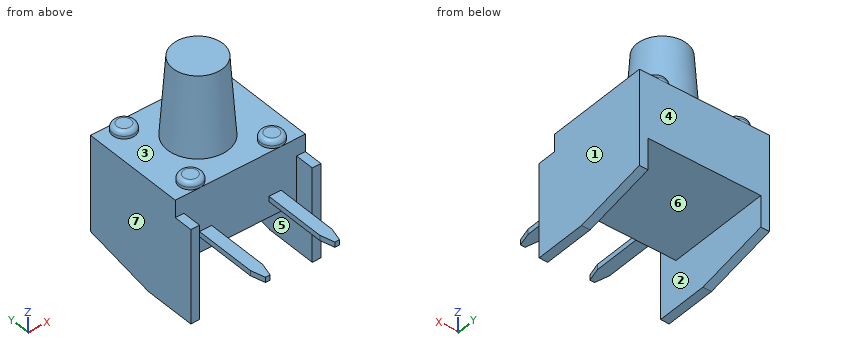
from build123d import *
from OCP.BRepFilletAPI import BRepFilletAPI_MakeChamfer

# Parameters (mm, degrees)
SKETCH1_W           = 7.5
SKETCH1_H           = 3.7
BOSS_EXTRUDE1_DEPTH = 6
SKETCH2_R           = 1.75
BOSS_EXTRUDE2_DEPTH = 4.5
BOSS_EXTRUDE2_TAPER = 4
SKETCH3_W           = 0.7
SKETCH3_H           = 0.3
BOSS_EXTRUDE3_DEPTH = 4.4
SKETCH4_W           = 0.5
SKETCH4_H           = 2.7
BOSS_EXTRUDE4_DEPTH = 1.1
BOSS_EXTRUDE5_DEPTH = 2.7
CUT_EXTRUDE1_DEPTH  = 12.541663658
SKETCH7_R           = 0.65
BOSS_EXTRUDE6_DEPTH = 0.4
FILLET1_R           = 0.25
CHAMFER1_SIZE       = 0.8
CHAMFER1_SIZE2      = 0.214359354


with BuildPart() as part:
    # Sketch1 → Boss-Extrude1 (new body)
    with BuildSketch(Plane(origin=(0, 0, 0), x_dir=(1, 0, 0), z_dir=(0, 1, 0))):
        with Locations((3.75, 1.85)):
            Rectangle(SKETCH1_W, SKETCH1_H)
    extrude(amount=BOSS_EXTRUDE1_DEPTH)

    # Sketch2 → Boss-Extrude2 (add)
    with BuildSketch(Plane.XY):
        with Locations((3.75, 3)):
            Circle(SKETCH2_R)
    extrude(amount=BOSS_EXTRUDE2_DEPTH, taper=BOSS_EXTRUDE2_TAPER)

    # Sketch3 → Boss-Extrude3 (add)
    with BuildSketch(Plane.XZ):
        with Locations((1.75, -2.65)):
            Rectangle(SKETCH3_W, SKETCH3_H)
        with Locations((5.75, -2.65)):
            Rectangle(SKETCH3_W, SKETCH3_H)
    extrude(amount=BOSS_EXTRUDE3_DEPTH)

    # Sketch4 → Boss-Extrude4 (add)
    with BuildSketch(Plane.XZ):
        with Locations((0.25, -2.35)):
            Rectangle(SKETCH4_W, SKETCH4_H)
        with Locations((7.25, -2.35)):
            Rectangle(SKETCH4_W, SKETCH4_H)
    extrude(amount=BOSS_EXTRUDE4_DEPTH)

    # Sketch5 → Boss-Extrude5 (add)
    with BuildSketch(Plane(origin=(0, 0, -3.7), x_dir=(-1, 0, 0), z_dir=(0, 0, -1))):
        Polygon((-7, 0), (-7, 6), (-7.5, 6), (-7.5, -1.1), (-7, -1.1), align=None)
        Polygon((-0.5, -1.1), (-0.5, 0), (-0.5, 6), (0, 6), (0, -1.1), align=None)
    extrude(amount=BOSS_EXTRUDE5_DEPTH)

    # Sketch6 → Cut-Extrude1 (cut, through all)
    with BuildSketch(Plane(origin=(7.5, 0, 0), x_dir=(0, 0, -1), z_dir=(1, 0, 0))):
        Polygon((5.5, 6), (6.4, 1.9), (6.4, 6), align=None)
    extrude(amount=-CUT_EXTRUDE1_DEPTH, mode=Mode.SUBTRACT)

    # Sketch7 → Boss-Extrude6 (add)
    with BuildSketch(Plane.XY):
        with Locations(Location((1.4, 5.35, 0), (0, 0, 90))):
            Circle(SKETCH7_R)
        with Locations(Location((6.1, 5.35, 0), (0, 0, 90))):
            Circle(SKETCH7_R)
        with Locations(Location((6.1, 0.65, 0), (0, 0, 270))):
            Circle(SKETCH7_R)
        with Locations(Location((1.4, 0.65, 0), (0, 0, 270))):
            Circle(SKETCH7_R)
    extrude(amount=BOSS_EXTRUDE6_DEPTH)

    # Fillet1
    fillet1_edges = [part.edges().sort_by_distance(p)[0] for p in [
        (1.4, 4.7, 0.4),
        (6.1, 4.7, 0.4),
        (6.1, 1.3, 0.4),
        (1.4, 1.3, 0.4),
    ]]
    fillet(fillet1_edges, radius=FILLET1_R)

    # Chamfer1: one chamfer whose edges measure the first distance from different faces: ONE call of the kernel's chamfer builder (chamfer() names one face for all edges)
    chamfer1_edges_1 = [part.edges().sort_by_distance(p)[0] for p in [
        (1.4, -4.4, -2.65),
    ]]
    chamfer1_side_1 = [part.faces().sort_by_distance(p)[0] for p in [
        (1.4, -2.2, -2.65),
    ]]
    chamfer1_edges_2 = [part.edges().sort_by_distance(p)[0] for p in [
        (2.1, -4.4, -2.65),
    ]]
    chamfer1_side_2 = [part.faces().sort_by_distance(p)[0] for p in [
        (2.1, -2.2, -2.65),
    ]]
    chamfer1_edges_3 = [part.edges().sort_by_distance(p)[0] for p in [
        (5.4, -4.4, -2.65),
    ]]
    chamfer1_side_3 = [part.faces().sort_by_distance(p)[0] for p in [
        (5.4, -2.2, -2.65),
    ]]
    chamfer1_edges_4 = [part.edges().sort_by_distance(p)[0] for p in [
        (6.1, -4.4, -2.65),
    ]]
    chamfer1_side_4 = [part.faces().sort_by_distance(p)[0] for p in [
        (6.1, -2.2, -2.65),
    ]]
    chamfer1 = BRepFilletAPI_MakeChamfer(part.part.solid().wrapped)
    for e in chamfer1_edges_1:
        chamfer1.Add(CHAMFER1_SIZE, CHAMFER1_SIZE2, e.wrapped, chamfer1_side_1[0].wrapped)  # the first distance lies on this face
    for e in chamfer1_edges_2:
        chamfer1.Add(CHAMFER1_SIZE, CHAMFER1_SIZE2, e.wrapped, chamfer1_side_2[0].wrapped)  # the first distance lies on this face
    for e in chamfer1_edges_3:
        chamfer1.Add(CHAMFER1_SIZE, CHAMFER1_SIZE2, e.wrapped, chamfer1_side_3[0].wrapped)  # the first distance lies on this face
    for e in chamfer1_edges_4:
        chamfer1.Add(CHAMFER1_SIZE, CHAMFER1_SIZE2, e.wrapped, chamfer1_side_4[0].wrapped)  # the first distance lies on this face
    add(Compound.cast(chamfer1.Shape()), mode=Mode.REPLACE)


solid = part.part
Geometry check sheet. Reference: the model listing, model coordinates, mm. Face numbers are marked on the shaded views. A direction names the side the tool comes from. Coordinates: 2 decimals unless noted, no trailing zeros. Loops run counter-clockwise (first coordinate to the right, second up) from the corner with the lowest first, then second, coordinate; pieces in that order, holes last. Notation, with made-up numbers: (14, -22.5) - (18, -22.5) arc R17 cw to (18, 4.5) - close; hole circle Ø7 at (0, 3). An arc over 180 degrees is marked (long way). Use one line per item in the form item = value. Start each with the question number.
Item 1: Section check C-C, the plane x = 3.75. Enter the section's corners in (y, z).
Item 2: Section check D-D, the plane y = 0.65. Enter the section's corners in (x, z).
Item 3: Gauge pin test, flat ends, axial feed: pin 1 (0.6 mm diameter, centred on x = 5.5, y = -1.5, fed in from -Z); pin 2 (1 mm diameter, centred on x = 6.5, y = 0.5, fed in from +Z); pin 3 (1.8 mm diameter, centred on x = 4, z = -1.5, fed in from -Y); pin 4 (2 mm diameter, centred on x = 4, z = -5, fed in from -Y). Record the tip position at first contact, or that the pin passes through.
Item 4: Thickness scan on probe 1 along X at (y, z) = (-2, -2.75); probe 2 along X at (y, z) = (2.75, -4.5); probe 3 along Z at (x, y) = (6.25, 1.75). Record the ranges inside material, lowest first.
Item 5: Section check B-B, the plane z = -2.25. Enter the section's corners in (x, y), and give its area (3 significant figures).
Item 6: Section check A-A, the plane y = -2. Enter the section's corners in (x, z), and give its area (3 significant figures).
Item 7: Mould release check, pull along X, two halves, no side actions. Record for the marked faces 4, 5, 6 and 7: +X half, -X half, draft (parallel to the pull), parting line (faces both ways), or undercut.
Item 8: Tool access check on the marked faces 1, 2 and 3. Record the directions out of +Z, -Z, +X, -X, +Y, -Y that give a thin tool (end or side, any length) a straight path to the whole face; none if there is none.
Computed:
q1.outline = (0, -3.7) - (6, -3.7) - (6, 0) - (4.75, 0) - (4.44, 4.5) - (1.56, 4.5) - (1.25, 0) - (0, 0) - close
q2.outline = (0, -6.4) - (0.5, -6.4) - (0.5, -3.7) - (7, -3.7) - (7, -6.4) - (7.5, -6.4) - (7.5, 0) - (6.75, 0) - (6.75, 0.15) arc R0.25 ccw to (6.5, 0.4) - (5.7, 0.4) arc R0.25 ccw to (5.45, 0.15) - (5.45, 0) - (2.05, 0) - (2.05, 0.15) arc R0.25 ccw to (1.8, 0.4) - (1, 0.4) arc R0.25 ccw to (0.75, 0.15) - (0.75, 0) - (0, 0) - close
q3.pin_1 = -2.8
q3.pin_2 = 0.4
q3.pin_3 = 0
q3.pin_4 = through
q4.probe_1 = 1.4 to 2.1, 5.4 to 6.1
q4.probe_2 = 0 to 0.5, 7 to 7.5
q4.probe_3 = -3.7 to 0
q5.outline = (0, -1.1) - (0.5, -1.1) - (0.5, 0) - (7, 0) - (7, -1.1) - (7.5, -1.1) - (7.5, 6) - (0, 6) - close
q5.area = 46.1 mm2
q6.outline = (1.4, -2.8) - (2.1, -2.8) - (2.1, -2.5) - (1.4, -2.5) - close; (5.4, -2.8) - (6.1, -2.8) - (6.1, -2.5) - (5.4, -2.5) - close
q6.area = 0.420 mm2
q7.face_4 = draft
q7.face_5 = undercut
q7.face_6 = undercut
q7.face_7 = -X half
q8.face_1 = +Z, -Z, +X, +Y, -Y
q8.face_2 = -Z, -Y
q8.face_3 = +Z
